Check sheet for the modelled part. Datum: model origin and axes. Units: mm. A direction names the side the tool comes from. Round coordinates to 2 decimals unless told otherwise and drop trailing zeros. Order: outer loops, then holes, each group sorted by start corner. A loop starts at its lowest first (then second) coordinate and runs counter-clockwise, first axis right, second up.
```python
from build123d import *

# Parameters (mm, degrees)
SKETCH1_R           = 101.6
BOSS_EXTRUDE1_DEPTH = 539.75
SKETCH2_R           = 31.75
BOSS_EXTRUDE2_DEPTH = 152.4
SKETCH3_R           = 63.5
BOSS_EXTRUDE3_DEPTH = 76.2


with BuildPart() as part:
    # Sketch1 → Boss-Extrude1 (new, symmetric)
    with BuildSketch(Plane(origin=(0, 0, 0), x_dir=(0, 0, -1), z_dir=(1, 0, 0))):
        Circle(SKETCH1_R)
    extrude(amount=BOSS_EXTRUDE1_DEPTH, both=True)

    # Sketch2 → Boss-Extrude2 (add, symmetric)
    with BuildSketch(Plane(origin=(0, 0, 0), x_dir=(1, 0, 0), z_dir=(0, 1, 0))):
        with Locations(Location((-476.25, 0, 0), (0, 0, 90))):
            Circle(SKETCH2_R)
    extrude(amount=BOSS_EXTRUDE2_DEPTH, both=True)

    # Sketch3 → Boss-Extrude3 (add)
    with BuildSketch(Plane.ZY.offset(539.75)):
        with Locations(Location((0, 0, 0), (0, 0, 180))):
            Circle(SKETCH3_R)
    extrude(amount=BOSS_EXTRUDE3_DEPTH)


solid = part.part
```
Item 1: Sectioned sample at B-B (z = 0). Record the cut outline in (x, y).
Answer:
outline: (-615.95, -63.5) - (-539.75, -63.5) - (-539.75, -101.6) - (-508, -101.6) - (-508, -152.4) - (-444.5, -152.4) - (-444.5, -101.6) - (539.75, -101.6) - (539.75, 101.6) - (-444.5, 101.6) - (-444.5, 152.4) - (-508, 152.4) - (-508, 101.6) - (-539.75, 101.6) - (-539.75, 63.5) - (-615.95, 63.5) - close
Item 2: Sectioned sample at D-D (x = 49.5). Record the cut outline in (y, z).
Answer:
outline: circle Ø203.2 at (0, 0)
Item 3: Sectioned sample at C-C (y = 0). Record the cut outline in (x, z), and give its area (3 significant figures).
Answer:
outline: (-615.95, -63.5) - (-539.75, -63.5) - (-539.75, -101.6) - (539.75, -101.6) - (539.75, 101.6) - (-539.75, 101.6) - (-539.75, 63.5) - (-615.95, 63.5) - close
area: 229,000 mm2
Item 4: Go/stop test with flat-tipped pins: P1, Ø10, axis at x = -447, z = -46.5, coming from the -Y side; P2, Ø12, axis at x = -451, y = 80, coming from the -Z side; P3, Ø8, axis at x = -471, y = 50, coming from the +Z side. Record where each tip stops, or that it passes through.
Answer:
P1: stops at y = -92.74
P2: stops at z = -69.62
P3: stops at z = 90.59
Item 5: Scan lines: line 1 along X through (y, z) = (-50.5, 80); line 2 along Z through (x, y) = (155, -6); line 3 along Y through (x, z) = (294, -32). Record each from-to range of solid material in increasing order.
Answer:
line 1: x = -539.75 to 539.75
line 2: z = -101.42 to 101.42
line 3: y = -96.43 to 96.43
Item 6: Access from +Z, -Z, +X, -X, +Y, -Y to the whole of each face (thin tool, end or side, straight path). Record for faces 1 (the flat face through (-615.95, -1, 1)), 2 (the cylindrical face through (-477.65, 124.85, 31.72)), 3 (the cylindrical face through (-577.32, 61.99, 13.77)), 4 (the cylindrical face through (-477.65, -124.06, 31.72)).
Answer:
face 1: +Z, -Z, -X, +Y, -Y
face 2: +Y
face 3: -X
face 4: -Y
Item 7: Sectioned sample at A-A (x = -476.25). Record the cut outline in (y, z), and give its area (3 significant figures).
Answer:
outline: (-152.4, -31.75) - (-96.51, -31.75) arc R101.6 ccw to (96.51, -31.75) - (152.4, -31.75) - (152.4, 31.75) - (96.51, 31.75) arc R101.6 ccw to (-96.51, 31.75) - (-152.4, 31.75) - close
area: 39,100 mm2
